Part model, mm, in its own coordinate system. A direction names the side the tool comes from. Round coordinates to 2 decimals unless told otherwise and drop trailing zeros. Loops run counter-clockwise (first coordinate to the right, second up) from the corner with the lowest first, then second, coordinate; pieces in that order, holes last. Notation, with made-up numbers: (75, 52) -> (125, 52) arc R22 cw to (125, 74) -> close; hole circle Ø4 at (-3, 16). An arc over 180 degrees is marked (long way). Answer as CSV lines item,"result".
from build123d import *

# Parameters (mm, degrees)
SKETCH1_W           = 50.8
SKETCH1_H           = 88.9
SKETCH1_R           = 1.5875
BOSS_EXTRUDE1_DEPTH = 3.175
SKETCH2_W           = 3.175
SKETCH2_H           = 50.8
CUT_EXTRUDE1_DEPTH  = 52.293694788
LPATTERN1_COUNT     = 3
LPATTERN1_PITCH     = 9.525
LPATTERN1_COL_COUNT = 3
LPATTERN1_COL_PITCH = 9.525
CUT_EXTRUDE2_DEPTH  = 52.293694788


with BuildPart() as part:
    # Sketch1 → Boss-Extrude1 (new body)
    with BuildSketch(Plane.XY):
        Rectangle(SKETCH1_W, SKETCH1_H)
        with Locations((-14.715789726, 25.75263202)):
            Circle(SKETCH1_R, mode=Mode.SUBTRACT)
    extrude(amount=BOSS_EXTRUDE1_DEPTH)

    # Sketch2 → Cut-Extrude1 (cut, through all)
    with BuildSketch(Plane.XY.offset(3.175)):
        with Locations((0, -19.05)):
            Rectangle(SKETCH2_W, SKETCH2_H)
    cut_extrude1 = extrude(amount=-CUT_EXTRUDE1_DEPTH, mode=Mode.SUBTRACT)

    # LPattern1: Cut-Extrude1 ×3
    with Locations(*[(i * LPATTERN1_PITCH, 0, 0) for i in range(1, LPATTERN1_COUNT)]):
        add(cut_extrude1, mode=Mode.SUBTRACT)

    # LPattern1 col: Cut-Extrude1 ×3
    with Locations(*[(-i * LPATTERN1_COL_PITCH, 0, 0) for i in range(1, LPATTERN1_COL_COUNT)]):
        add(cut_extrude1, mode=Mode.SUBTRACT)

    # Sketch3 → Cut-Extrude2 (cut, through all)
    with BuildSketch(Plane.XY.offset(3.175)):
        Polygon((-11.1379, 6.3754), (-11.1379, -44.45), (-11.1125, -44.45), (-11.1125, 6.35), (-7.9375, 6.35), (-7.9375, -44.45), (-7.9121, -44.45), (-7.9121, 6.3754), align=None)
        Polygon((-1.6383, 6.4008), (-1.6383, -44.45), (-1.5875, -44.45), (-1.5875, 6.35), (1.5875, 6.35), (1.5875, -44.45), (1.6383, -44.45), (1.6383, 6.4008), align=None)
        Polygon((7.8613, 6.4262), (7.8613, -44.45), (7.9375, -44.45), (7.9375, 6.35), (11.1125, 6.35), (11.1125, -44.45), (11.1887, -44.45), (11.1887, 6.4262), align=None)
        Polygon((20.6375, -44.45), (20.7391, -44.45), (20.7391, 6.4516), (17.3609, 6.4516), (17.3609, -44.45), (17.4625, -44.45), (17.4625, 6.35), (20.6375, 6.35), align=None)
    extrude(amount=-CUT_EXTRUDE2_DEPTH, mode=Mode.SUBTRACT)


solid = part.part
Q1. Saw through at C-C, the plane x = 0. Write the cut outline in (y, z) (3 decimals), then the cut area to 3 significant figures.
Geometry results:
outline,"(6.401, 0) -> (44.45, 0) -> (44.45, 3.175) -> (6.401, 3.175) -> close"
area,"121 mm2"
Q2. Drill centre lines: line 1 along X through (y, z) = (-23, 2.35); line 2 along Y through (x, z) = (8.5, 0.9); line 3 along Y through (x, z) = (-16, 0.7). Where is each one in solid material? Low to high.
Geometry results:
line 1,"-25.4 to -20.64, -17.46 to -11.14, -7.91 to -1.64, 1.64 to 7.86, 11.19 to 17.36, 20.74 to 25.4"
line 2,"6.43 to 44.45"
line 3,"-44.45 to 24.82, 26.69 to 44.45"
Q3. Which spindle directions (+Z, -Z, +X, -X, +Y, -Y) get a long thin tool onto all of the face, cutting with end or side? Do faces 4 (the face through (1.638, -19, 2)), 5 (the face through (0, 44.45, 2)). Say none if no direction does.
Geometry results:
face 4,"+Z, -Z, -Y"
face 5,"+Z, -Z, +X, -X, +Y"
Q4. Saw through at A-A, the plane y = -20.5. Write the cut outline in (x, z) (1 decimal), then the cut area to 3 significant figures.
Geometry results:
outline,"(-25.4, 0) -> (-20.6, 0) -> (-20.6, 3.2) -> (-25.4, 3.2) -> close; (-17.5, 0) -> (-11.1, 0) -> (-11.1, 3.2) -> (-17.5, 3.2) -> close; (-7.9, 0) -> (-1.6, 0) -> (-1.6, 3.2) -> (-7.9, 3.2) -> close; (1.6, 0) -> (7.9, 0) -> (7.9, 3.2) -> (1.6, 3.2) -> close; (11.2, 0) -> (17.4, 0) -> (17.4, 3.2) -> (11.2, 3.2) -> close; (20.7, 0) -> (25.4, 0) -> (25.4, 3.2) -> (20.7, 3.2) -> close"
area,"109 mm2"
Q5. Drop flat-ended pins along their axis: P1, Ø1, axis at x = -9.5, z = 1, coming from the -Y side; P2, Ø1, axis at x = -20, z = 2, coming from the -Y side. Give the stop position or say it passes through.
Geometry results:
P1,"y = 6.38"
P2,"y = 6.35"
Q6. Two-plate mould, pull along X, no slides. Class faces 1 (the face through (-5, -44.45, 2)), 2 (the face through (20.739, -19, 2)), 3 (the face through (25.4, -1, 2)): pulls with the +X half, pulls with the -X half, needs draft (parallel to the pull), parting line crosses it, or undercut.
Geometry results:
face 1,"needs draft"
face 2,"undercut"
face 3,"pulls with the +X half"
